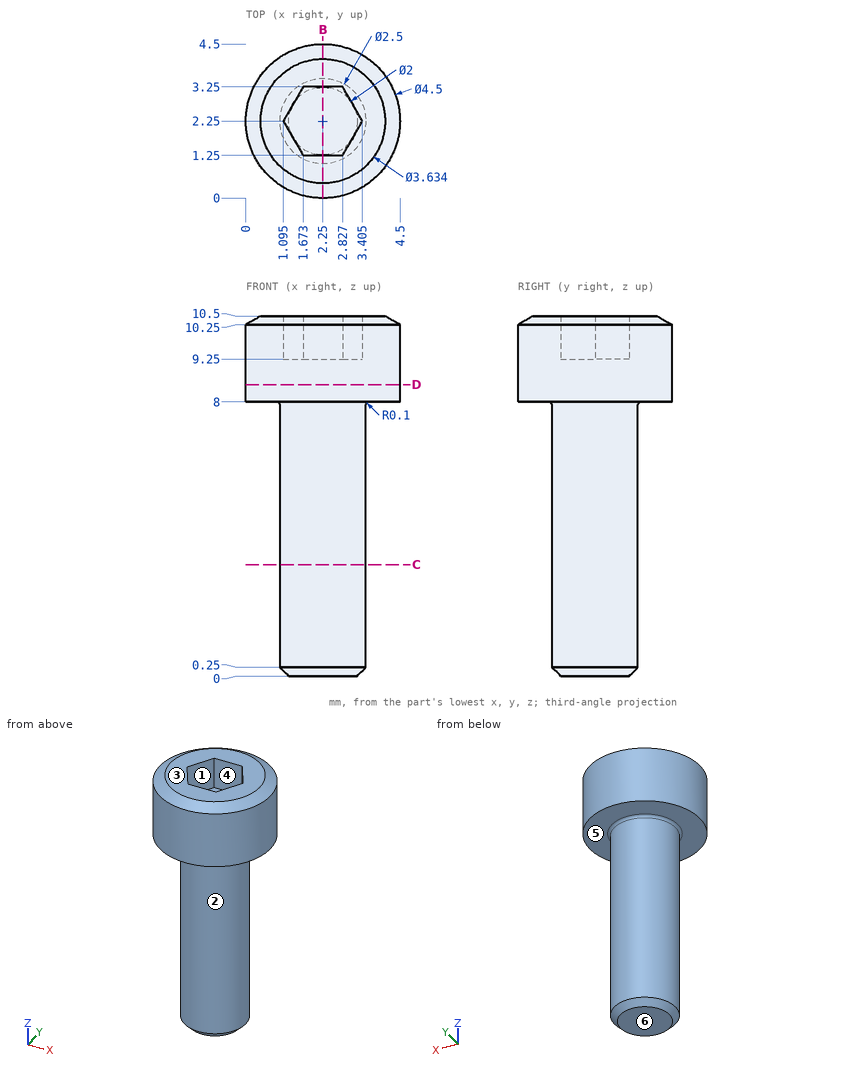
Print and shaded views of the part. All mm, measured from the part's lowest x, y and z. A direction names the side the tool comes from. Coordinates: 2 decimals unless noted, no trailing zeros. Write each loop counter-clockwise with the first axis right and the second up, starting at its lowest first coordinate (ties: lowest second). Pieces come first, ordered by that corner, then holes.
(1) 3-axis set-ups, long thin cutter, end or side, ignore diameter. For the marked faces 4, 5 and 6: which of +Z, -Z, +X, -X, +Y, -Y reach the whole face in a straight line?
(2) Cut at C-C, the plane z = 3.25. List the corners of the cut face in (x, y).
(3) Cut at B-B, the plane x = 2.25. List the corners of the cut face in (y, z).
(4) Cut at D-D, the plane z = 8.5. List the corners of the cut face in (x, y).
(5) Drill centre lines: probe 1 along Z at (x, y) = (2.4, 2.9); probe 2 along Z at (x, y) = (0.95, 1.45); probe 3 along Y at (x, z) = (2, 9.5). Where is each one in solid material? Low to high.
(6) Flat gauge pins, fed straight in: pin 1 (1 mm diameter, centred on x = 1.5, z = 6, fed in from -Y) (1 decimal); pin 2 (1 mm diameter, centred on x = 2, y = 2, fed in from +Z); pin 3 (1.3 mm diameter, centred on x = 1.5, y = 2, fed in from -Z). Where does each tip first touch, or does it go through?
(7) Two-plate mould, pull along Y, no slides. Class the marked faces 1, 2 and 3: +Y half, -Y half, draft (parallel to the pull), parting line (faces both ways), or undercut.
Geometry says:
1. face 4: +Z
1. face 5: -Z
1. face 6: -Z, +X, -X, +Y, -Y
2. outline: circle Ø2.5 at (2.25, 2.25)
3. outline: (0, 8) - (0.9, 8) arc R0.1 cw to (1, 7.9) - (1, 0.25) - (1.25, 0) - (3.25, 0) - (3.5, 0.25) - (3.5, 7.9) arc R0.1 cw to (3.6, 8) - (4.5, 8) - (4.5, 10.25) - (4.07, 10.5) - (3.25, 10.5) - (3.25, 9.25) - (1.25, 9.25) - (1.25, 10.5) - (0.43, 10.5) - (0, 10.25) - close
4. outline: circle Ø4.5 at (2.25, 2.25)
5. probe 1: z = 0 to 9.25
5. probe 2: z = 8 to 10.5
5. probe 3: y = 0.01 to 1.25, 3.25 to 4.49
6. pin 1: stops at y = 1
6. pin 2: stops at z = 9.25
6. pin 3: stops at z = 0
7. face 1: undercut
7. face 2: parting line
7. face 3: draft
